Can you work these out from the model? Positions are in its coordinate system, mm. A direction names the side the tool comes from. Coordinates: 2 decimals unless noted, no trailing zeros. Loops run counter-clockwise (first coordinate to the right, second up) from the corner with the lowest first, then second, coordinate; pieces in that order, holes last.
```python
from build123d import *

# Parameters (mm, degrees)
F_1_2_13_TAPPED_HOLE1_D     = 10.71626
BOSS_EXTRUDE1_START         = -8.5
SKETCH9_W                   = 45
SKETCH9_H                   = 28
SKETCH9_R                   = 13.5
BOSS_EXTRUDE1_DEPTH         = 8.5
TAP_DRILL_FOR_M5X0_8_TAP1_D = 4.2
FILLET1_R                   = 9
CHAMFER1_SIZE               = 1
SKETCH8_R                   = 11.5
CUT_EXTRUDE2_DEPTH          = 12


with BuildPart() as part:
    # Sketch2 → Revolve1 (revolve)
    with BuildSketch(Plane(origin=(0, 0, 0), x_dir=(0, 0, -1), z_dir=(1, 0, 0)), mode=Mode.PRIVATE) as revolve1_sk:
        Polygon((0, 13.5), (16.9, 13.5), (16.9, 14), (25.4, 14), (25.4, 0), (0, 0), align=None)
    revolve(revolve1_sk.sketch.rotate(Axis((0, 0, 0), (0, 0, 1)), 90), axis=Axis((0, 0, 0), (0, 0, 1)))

    # 1/2-13 Tapped Hole1 (through all)
    with Locations(Plane.XY):
        with Locations((0, 0)):
            Hole(F_1_2_13_TAPPED_HOLE1_D / 2)

    # Sketch9 → Boss-Extrude1 (add)
    with BuildSketch(Plane.XY.offset(-16.9).offset(BOSS_EXTRUDE1_START)):
        Rectangle(SKETCH9_W, SKETCH9_H)
        with Locations(Location((0, 0, 0), (0, 0, 180))):
            Circle(SKETCH9_R, mode=Mode.SUBTRACT)
    extrude(amount=BOSS_EXTRUDE1_DEPTH)

    # Tap Drill for M5x0.8 Tap1 (through all)
    with Locations(Plane.XY.offset(-16.9)):
        with Locations((-19, 0), (19, 0)):
            Hole(TAP_DRILL_FOR_M5X0_8_TAP1_D / 2)

    # Fillet1
    fillet1_edges = [part.edges().sort_by_distance(p)[0] for p in [
        (-22.5, 14, -21.15),
        (22.5, -14, -21.15),
        (-22.5, -14, -21.15),
        (22.5, 14, -21.15),
    ]]
    fillet(fillet1_edges, radius=FILLET1_R)

    # Chamfer1
    chamfer1_edges = [part.edges().sort_by_distance(p)[0] for p in [
        (13.5, 0, 0),
    ]]
    chamfer(chamfer1_edges, length=CHAMFER1_SIZE)

    # Sketch8 → Cut-Extrude2 (cut)
    with BuildSketch(Plane(origin=(0, 0, -25.4), x_dir=(-1, 0, 0), z_dir=(0, 0, -1))):
        Circle(SKETCH8_R)
    extrude(amount=-CUT_EXTRUDE2_DEPTH, mode=Mode.SUBTRACT)


solid = part.part
```
(1) Which directions (+Z, -Z, +X, -X, +Y, -Y) give clear straight access to the entire face, cutting with the end or side of a thin tool? Please do faces 4 (the flat face through (0, -14, -21)), 5 (the cylindrical face through (1.5, 11.4, -19.5)), 6 (the cylindrical face through (2.93, 13.18, -9.06)).
Check values:
face 4: +Z, -Z, +X, -X, -Y
face 5: -Z
face 6: +Z
(2) I want a section at A-A on x = -19. Write out the boundary of the cut face in (y, z).
Check values:
outline: (-12.12, -25.4) - (-2.1, -25.4) - (-2.1, -16.9) - (-12.12, -16.9) - close; (2.1, -25.4) - (12.12, -25.4) - (12.12, -16.9) - (2.1, -16.9) - close
(3) I want a section at D-D on x = 18.5. Write out the boundary of the cut face in (y, z), then the cut area to 3 significant figures.
Check values:
outline: (-12.48, -25.4) - (-2.04, -25.4) - (-2.04, -16.9) - (-12.48, -16.9) - close; (2.04, -25.4) - (12.48, -25.4) - (12.48, -16.9) - (2.04, -16.9) - close
area: 178 mm2
(4) If we mould it in two halves opening along Y, with no side actions, what happens to faces 1 (the cylindrical face through (-19.934, -11.294, -21.09)), 2 (the cylindrical face through (-19.934, 11.294, -21.09)), 3 (the flat face through (-5, -2.4, -13.4))? For each: released by +Y, released by -Y, zero draft, split by the parting line, or undercut.
Check values:
face 1: released by -Y
face 2: released by +Y
face 3: undercut
(5) I want a section at C-C on z = -14. Write out the boundary of the cut face in (x, y).
Check values:
outline: circle Ø27 at (0, 0); hole circle Ø23 at (0, 0)
(6) I'm going to push flat-ended pins straight in: pin 1 (1 mm diameter, centred on y = 0.5, z = -8, fed in from +X); pin 2 (1 mm diameter, centred on y = 5.5, z = -19, fed in from +X); pin 3 (7 mm diameter, centred on x = -5.5, y = 2, fed in from -Z); pin 4 (10 mm diameter, centred on x = 11.5, z = -3, fed in from +Y). Where does each tip first touch, or does it pass through?
Check values:
pin 1: stops at x = 13.5
pin 2: stops at x = 22.5
pin 3: stops at z = -13.4
pin 4: stops at y = 11.83
(7) If I drill on probe 1 along Y at (x, z) = (0, -9.25); probe 2 along Z at (x, y) = (5, -3.5); probe 3 along Y at (x, z) = (-2, -13.75), over which ranges is the centre line in solid material (lowest first)?
Check values:
probe 1: y = -13.5 to -5.36, 5.36 to 13.5
probe 2: z = -13.4 to 0
probe 3: y = -13.35 to -11.32, 11.32 to 13.35
(8) I want a section at B-B on z = -5.25. Write out the boundary of the cut face in (x, y), then the cut area to 3 significant figures.
Check values:
outline: circle Ø27 at (0, 0); hole circle Ø10.72 at (0, 0)
area: 482 mm2
